```python
from build123d import *
from OCP.BRepAlgoAPI import BRepAlgoAPI_Cut
from OCP.TopTools import TopTools_ListOfShape

# Parameters (mm, degrees)
SZKIC1_W                               = 25
SZKIC1_H                               = 20
DODANIE_WYCI_GNI_CIE1_DEPTH            = 42.5
WYTNIJ_WYCI_GNI_CIE1_REACH             = 52.312
SZKIC2_R                               = 5.1
WYTNIJ_WYCI_GNI_CIE2_REACH             = 50.606
SZKIC3_R                               = 5.1
DODANIE_WYCI_GNI_CIE2_START            = -20
DODANIE_WYCI_GNI_CIE2_DEPTH            = 20
ZAOKR_GLENIE2_R                        = 0.75
SZKIC7_W                               = 25
SZKIC7_H                               = 15
DODANIE_WYCI_GNI_CIE3_DEPTH            = 2
WYTNIJ_WYCI_GNI_CIE4_REACH             = 49.817
SZKIC8_R                               = 4.05
SFAZOWANIE1_SIZE                       = 7.5
WYCI_CIE_WYCI_GNI_CIE_START            = 5.5
WYCI_CIE_WYCI_GNI_CIE_PO_CIE_CE1_DEPTH = 3
ZAOKR_GLENIE3_R                        = 2
ZAOKR_GLENIE4_START                    = -11
ZAOKR_GLENIE4_DEPTH                    = 22
ZAOKR_GLENIE3_OF_LUSTRO2_R             = 2
ZAOKR_GLENIE5_R                        = 5
ZAOKR_GLENIE6_R                        = 1
SFAZOWANIE2_SIZE                       = 1.5
WYTNIJ_WYCI_GNI_CIE5_REACH             = 52.312
SZKIC12_R                              = 5.1


with BuildPart() as part:
    # Szkic1 → Dodanie-wyciągnięcie1 (new body)
    with BuildSketch(Plane.XY):
        Rectangle(SZKIC1_W, SZKIC1_H)
    extrude(amount=DODANIE_WYCI_GNI_CIE1_DEPTH)

    # Szkic2 → Wytnij-wyciągnięcie1 (cut, up to next)
    with BuildSketch(Plane(origin=(12.5, 0, 0), x_dir=(0, 0, -1), z_dir=(1, 0, 0)), mode=Mode.PRIVATE) as wytnij_wyci_gni_cie1_sk1:
        with Locations((-8, 0)):
            Circle(SZKIC2_R)
    wytnij_wyci_gni_cie1_tool1 = extrude(wytnij_wyci_gni_cie1_sk1.sketch, amount=-WYTNIJ_WYCI_GNI_CIE1_REACH, mode=Mode.PRIVATE) & part.part
    add(wytnij_wyci_gni_cie1_tool1.solids().sort_by_distance((12.5, 0, 8))[0], mode=Mode.SUBTRACT)

    # Szkic3 → Wytnij-wyciągnięcie2 (cut, up to next)
    with BuildSketch(Plane(origin=(0, 10, 0), x_dir=(1, 0, 0), z_dir=(0, 1, 0)), mode=Mode.PRIVATE) as wytnij_wyci_gni_cie2_sk1:
        with Locations(Location((0, -19.5, 0), (0, 0, 270))):
            Circle(SZKIC3_R)
    wytnij_wyci_gni_cie2_tool1 = extrude(wytnij_wyci_gni_cie2_sk1.sketch, amount=-WYTNIJ_WYCI_GNI_CIE2_REACH, mode=Mode.PRIVATE) & part.part
    add(wytnij_wyci_gni_cie2_tool1.solids().sort_by_distance((0, 10, 19.5))[0], mode=Mode.SUBTRACT)

    # Dodanie-wyciągnięcie2: read off the stored shape, not the designer's step
    # Dodanie-wyciągnięcie2 outline → Dodanie-wyciągnięcie2 (add)
    with BuildSketch(Plane(origin=(0, 10, 0), x_dir=(1, 0, 0), z_dir=(0, 1, 0)).offset(DODANIE_WYCI_GNI_CIE2_START)):
        with BuildLine():
            Line((-12.5, 0), (-2.545584412, 0))
            ThreePointArc((-2.545584412, 0), (-4.049799766, 3.19027229), (-2.482438317, 6.35))
            Line((-2.482438317, 6.35), (-12.5, 6.35))
            Line((-12.5, 6.35), (-12.5, 0))
        make_face()
        with BuildLine():
            Line((12.5, 0), (12.5, 6.35))
            Line((12.5, 6.35), (2.482438317, 6.35))
            ThreePointArc((2.482438317, 6.35), (4.049799766, 3.19027229), (2.545584412, 0))
            Line((2.545584412, 0), (12.5, 0))
        make_face()
    extrude(amount=DODANIE_WYCI_GNI_CIE2_DEPTH)

    # Zaokrąglenie2
    zaokr_glenie2_edges = [part.edges().sort_by_distance(p)[0] for p in [
        (-2.482438317, 0, -6.35),
        (2.482438317, 0, -6.35),
    ]]
    fillet(zaokr_glenie2_edges, radius=ZAOKR_GLENIE2_R)

    # Szkic7 → Dodanie-wyciągnięcie3 (add)
    with BuildSketch(Plane.XZ.offset(10)):
        with Locations((0, 1.15)):
            Rectangle(SZKIC7_W, SZKIC7_H)
    extrude(amount=-DODANIE_WYCI_GNI_CIE3_DEPTH)

    # Szkic8 → Wytnij-wyciągnięcie4 (cut, up to next)
    with BuildSketch(Plane(origin=(0, -8, 0), x_dir=(1, 0, 0), z_dir=(0, 1, 0)), mode=Mode.PRIVATE) as wytnij_wyci_gni_cie4_sk1:
        with Locations((0, 3.15)):
            Circle(SZKIC8_R)
    wytnij_wyci_gni_cie4_tool1 = extrude(wytnij_wyci_gni_cie4_sk1.sketch, amount=WYTNIJ_WYCI_GNI_CIE4_REACH, mode=Mode.PRIVATE) & part.part
    add(wytnij_wyci_gni_cie4_tool1.solids().sort_by_distance((0, -8, -3.15))[0], mode=Mode.SUBTRACT)

    # Sfazowanie1
    sfazowanie1_edges = [part.edges().sort_by_distance(p)[0] for p in [
        (-12.5, 0, -6.35),
        (12.5, 0, -6.35),
    ]]
    chamfer(sfazowanie1_edges, length=SFAZOWANIE1_SIZE)


with BuildPart() as wyci_cie_wyci_gni_cie_po_cie_ce1_tool:
    # Wycięcie-wyciągnięcie po ścieżce1: read off the stored shape, not the designer's step
    # Wycięcie-wyciągnięcie po ścieżce1 outlin → Wycięcie-wyciągnięcie po ścieżce1 (new body)
    with BuildSketch(Plane(origin=(0, 0, 0), x_dir=(1, 0, 0), z_dir=(0, 1, 0)).offset(WYCI_CIE_WYCI_GNI_CIE_START)):
        with BuildLine():
            Line((-8.398959236, 2.951040764), (-9.601040764, 1.748959236))
            add(Edge.make_bspline(
                [(-9.601040764, 1.748959236), (-9.209595956, 0.772190109), (-8.65567701, -0.205079485), (-7.121419805, -2.018854383), (-6.15542851, -2.840889353), (-3.89496705, -4.097344098), (-2.618886758, -4.525976788), (0.018436022, -4.858092268), (1.356613032, -4.766181401), (3.844325913, -4.116700841), (4.978679647, -3.572124587), (6.907257886, -2.213562211), (7.697476445, -1.410485572), (8.875702434, 0.189942932), (9.295310391, 0.978883557), (9.600922152, 1.74907375)],
                knots=[0.044527741, 0.044527741, 0.044527741, 0.044527741, 0.163961774, 0.163961774, 0.283395806, 0.283395806, 0.402829838, 0.402829838, 0.522263871, 0.522263871, 0.641697903, 0.641697903, 0.761131935, 0.761131935, 0.869411924, 0.869411924, 0.869411924, 0.869411924], degree=3))
            Line((9.600922152, 1.74907375), (8.398612397, 2.951387603))
            add(Edge.make_bspline(
                [(-8.398959236, 2.951040764), (-8.143623085, 2.110383322), (-7.721254142, 1.22892436), (-6.543030407, -0.407961014), (-5.768609422, -1.171170966), (-3.942260695, -2.384057538), (-2.87593166, -2.830554933), (-0.670426419, -3.287743264), (0.481400093, -3.292782379), (2.627656604, -2.909796026), (3.631791424, -2.516326215), (5.35458893, -1.493813298), (6.079684963, -0.860499), (7.238136236, 0.482263814), (7.674817273, 1.192485201), (8.155489955, 2.24471168), (8.28334822, 2.593485223), (8.398612397, 2.951387603)],
                knots=[0.044527741, 0.044527741, 0.044527741, 0.044527741, 0.163961774, 0.163961774, 0.283395806, 0.283395806, 0.402829838, 0.402829838, 0.522263871, 0.522263871, 0.641697903, 0.641697903, 0.761131935, 0.761131935, 0.880565968, 0.880565968, 0.940774458, 0.940774458, 0.940774458, 0.940774458], degree=3))
        make_face()
    wyci_cie_wyci_gni_cie_po_cie_ce1 = extrude(amount=WYCI_CIE_WYCI_GNI_CIE_PO_CIE_CE1_DEPTH)


with BuildPart() as part_1:
    add(part.part)

    # Wycięcie-wyciągnięcie po ścieżce1: cut by wyci_cie_wyci_gni_cie_po_cie_ce1_tool, with a tolerance
    wyci_cie_wyci_gni_cie_po_cie_ce1_stock = TopTools_ListOfShape()
    wyci_cie_wyci_gni_cie_po_cie_ce1_stock.Append(part_1.part.wrapped)
    wyci_cie_wyci_gni_cie_po_cie_ce1_tools = TopTools_ListOfShape()
    wyci_cie_wyci_gni_cie_po_cie_ce1_tools.Append(wyci_cie_wyci_gni_cie_po_cie_ce1_tool.part.wrapped)
    wyci_cie_wyci_gni_cie_po_cie_ce1_cut = BRepAlgoAPI_Cut()
    wyci_cie_wyci_gni_cie_po_cie_ce1_cut.SetArguments(wyci_cie_wyci_gni_cie_po_cie_ce1_stock)
    wyci_cie_wyci_gni_cie_po_cie_ce1_cut.SetTools(wyci_cie_wyci_gni_cie_po_cie_ce1_tools)
    wyci_cie_wyci_gni_cie_po_cie_ce1_cut.SetFuzzyValue(0.00001)
    wyci_cie_wyci_gni_cie_po_cie_ce1_cut.Build()
    add(Compound.cast(wyci_cie_wyci_gni_cie_po_cie_ce1_cut.Shape()).solids(), mode=Mode.REPLACE)

    # Zaokrąglenie3
    zaokr_glenie3_edges = [part_1.edges().sort_by_distance(p)[0] for p in [
        (-8.398959236, 7, -2.951040764),
        (8.398612397, 7, -2.951387603),
    ]]
    fillet(zaokr_glenie3_edges, radius=ZAOKR_GLENIE3_R)

    # Zaokrąglenie4: read off the stored shape, not the designer's step
    # Zaokrąglenie4 outline → Zaokrąglenie4 (cut)
    with BuildSketch(Plane(origin=(0, 0, 0), x_dir=(1, 0, 0), z_dir=(0, 1, 0)).offset(ZAOKR_GLENIE4_START)):
        with BuildLine():
            Line((5, 6.35), (3.757359313, 6.35))
            ThreePointArc((3.757359313, 6.35), (4.90540961, 6.121638598), (5.878679656, 5.471320344))
            Line((5.878679656, 5.471320344), (5, 6.35))
        make_face()
        with BuildLine():
            ThreePointArc((-5.878679656, 5.471320344), (-4.90540961, 6.121638598), (-3.757359313, 6.35))
            Line((-3.757359313, 6.35), (-5, 6.35))
            Line((-5, 6.35), (-5.878679656, 5.471320344))
        make_face()
    extrude(amount=ZAOKR_GLENIE4_DEPTH, mode=Mode.SUBTRACT)

    # Lustro2: Wycięcie-wyciągnięcie po ścieżce1 across plane
    add(wyci_cie_wyci_gni_cie_po_cie_ce1.mirror(Plane.ZX), mode=Mode.SUBTRACT)

    # Zaokrąglenie3 of Lustro2
    zaokr_glenie3_of_lustro2_edges = [part_1.edges().sort_by_distance(p)[0] for p in [
        (-8.398959236, -7, -2.951040764),
        (8.398612397, -7, -2.951387603),
    ]]
    fillet(zaokr_glenie3_of_lustro2_edges, radius=ZAOKR_GLENIE3_OF_LUSTRO2_R)

    # Zaokrąglenie5
    # the kernel refuses this fillet: 5 mm, written as the material it takes off along each edge
    with BuildSketch(Plane(origin=(-12.5, 15.17766953, 1.15), x_dir=(0.7071067811865477, 0, -0.7071067811865472), z_dir=(0, -1, 0)), Plane(origin=(12.5, -15.17766953, 1.15), x_dir=(-0.7071067811865474, 0, -0.7071067811865476), z_dir=(0, 1, 0))) as zaokr_glenie5_piece_1:
        with BuildLine():
            CenterArc((ZAOKR_GLENIE5_R * 0.414213562373, ZAOKR_GLENIE5_R), ZAOKR_GLENIE5_R, 225, 45)
            Line((-ZAOKR_GLENIE5_R * 0.292893218813, ZAOKR_GLENIE5_R * 0.292893218813), (0, 0))
            Line((0, 0), (ZAOKR_GLENIE5_R * 0.414213562373, 0))
        make_face()
    extrude(amount=30.355339059, mode=Mode.SUBTRACT)

    # Zaokrąglenie6
    zaokr_glenie6_edges = [part_1.edges().sort_by_distance(p)[0] for p in [
        (-8.457106781, 10, -2.892893219),
        (-5.01866332, 10, -6.071968443),
        (5.01866332, 10, -6.071968443),
        (8.457106781, 10, -2.892893219),
        (12.119397663, 10, 1.30765065),
        (-12.119397663, 10, 1.30765065),
        (-12.5, 10, 22.860533906),
        (12.5, 10, 22.860533906),
    ]]
    fillet(zaokr_glenie6_edges, radius=ZAOKR_GLENIE6_R)

    # Sfazowanie2
    # the kernel refuses this chamfer: 1.5 mm, written as the material it takes off along each edge
    with BuildSketch(Plane(origin=(1e-09, 10, -3.15), x_dir=(0.08224322624349094, 0, -0.9966122875707795), z_dir=(-0.9966122875707795, 0, -0.08224322624349094))) as sfazowanie2_piece_1:
        Polygon((4.049999999 + SFAZOWANIE2_SIZE, 0), (4.049999999, SFAZOWANIE2_SIZE), (4.049999999, 0), align=None)
    revolve(axis=Axis((1e-09, 10, -3.15), (0, -1, 0)), revolution_arc=136.340040588, mode=Mode.SUBTRACT)
    with BuildSketch(Plane(origin=(-1e-09, 10, -3.15), x_dir=(-0.6285393608328834, 0, 0.7777777779570398), z_dir=(0.7777777779570398, 0, 0.6285393608328834))) as sfazowanie2_piece_2:
        Polygon((4.049999999 + SFAZOWANIE2_SIZE, 0), (4.049999999, SFAZOWANIE2_SIZE), (4.049999999, 0), align=None)
    revolve(axis=Axis((-1e-09, 10, -3.15), (0, -1, 0)), revolution_arc=136.340040588, mode=Mode.SUBTRACT)
    with BuildSketch(Plane(origin=(0, 10, -3.15), x_dir=(0.6285393610141453, 0, 0.7777777778105581), z_dir=(0.7777777778105581, 0, -0.6285393610141453))) as sfazowanie2_piece_3:
        Polygon((4.05 + SFAZOWANIE2_SIZE, 0), (4.05, SFAZOWANIE2_SIZE), (4.05, 0), align=None)
    revolve(axis=Axis((0, 10, -3.15), (0, -1, 0)), revolution_arc=77.884882532, mode=Mode.SUBTRACT)

    # Szkic12 → Wytnij-wyciągnięcie5 (cut, up to next)
    with BuildSketch(Plane.ZY.offset(12.5), mode=Mode.PRIVATE) as wytnij_wyci_gni_cie5_sk1:
        with Locations((32.5, 0)):
            Circle(SZKIC12_R)
    wytnij_wyci_gni_cie5_tool1 = extrude(wytnij_wyci_gni_cie5_sk1.sketch, amount=-WYTNIJ_WYCI_GNI_CIE5_REACH, mode=Mode.PRIVATE) & part_1.part
    add(wytnij_wyci_gni_cie5_tool1.solids().sort_by_distance((-12.5, 0, 32.5))[0], mode=Mode.SUBTRACT)


solid = part_1.part
```
CAD build for the part. Positions are in the model's coordinates, mm. A direction names the side the tool comes from. Round coordinates to 2 decimals unless told otherwise and drop trailing zeros. Order: outer loops, then holes, each group sorted by start corner. A loop starts at its lowest first (then second) coordinate and runs counter-clockwise, first axis right, second up. Notation, with made-up numbers: (-1.5, 16) - (29.5, 16) arc R29 ccw to (29.5, 41) - close; hole circle Ø5 at (87.25, 77). An arc over 180 degrees is marked (long way). Answer as CSV lines item,"result". Start each with the question number.
1. Saw through at D-D, the plane z = 19.5. Write the cut outline in (x, y).
2. Tool access for faces 5 (the face through (1.532, 0.14, 24.364)), 6 (the face through (0, 8.5, 3.4)), 7 (the face through (3.443, 0.809, -5.907)): list every direction of +Z, -Z, +X, -X, +Y, -Y with a clear straight run to the whole face (end or side of a thin tool).
3. Saw through at A-A, the plane z = 32.5. Write the cut outline in (x, y).
4. Pull direction X, two halves, no side cores. Call faces 1 (the face through (0, -8, -3)), 2 (the face through (12.5, -1, 23)), 3 (the face through (-12.215, 9.699, 23.135)), 4 (the face through (0, -9, -6.35)): +X half, -X half, draft (parallel to the pull), parting line (faces both ways), or undercut.
5. Saw through at B-B, the plane y = 3.5. Write the cut outline in (x, z), and give its area (3 significant figures).
6. Drill centre lines: L1, parallel to Y at x = 3.75, z = 8; L2, parallel to Z at x = -6, y = 0.25; L3, parallel to Z at x = -0.75, y = 2.5. Where is each one in solid material? Low to high. Write a range as [from, to].
7. Saw through at C-C, the plane x = 0. Count the separate pieces of the cut face and the enclosed holes in it, and give its area (3 significant figures).
8. Pin check, flat tips, straight feed: pin 1 (2 mm diameter, centred on x = 1.5, z = -1.5, fed in from +Y); pin 2 (11.5 mm diameter, centred on y = 0, z = 8, fed in from -X); pin 3 (4 mm diameter, centred on x = 9.5, y = 6, fed in from -Z); pin 4 (1.5 mm diameter, centred on x = 0, y = 1, fed in from -Z). Stop position of each tip, or through.
Model answer:
1,outline,"(-12.5, -10) - (-5.1, -10) - (-5.1, 10) - (-11.5, 10) arc R1 ccw to (-12.5, 9) - close; (5.1, -10) - (12.5, -10) - (12.5, 9) arc R1 ccw to (11.5, 10) - (5.1, 10) - close"
2,face 5,"+Y, -Y"
2,face 6,"none"
2,face 7,"+Y"
3,outline,"(-12.5, -10) - (12.5, -10) - (12.5, -5.1) - (-12.5, -5.1) - close; (-12.5, 5.1) - (12.5, 5.1) - (12.5, 9) arc R1 ccw to (11.5, 10) - (-11.5, 10) arc R1 ccw to (-12.5, 9) - close"
4,face 1,"undercut"
4,face 2,"+X half"
4,face 3,"-X half"
4,face 4,"draft"
5,outline,"(-12.5, 3.22) arc R5 ccw to (-11.04, -0.31) - (-5.88, -5.47) arc R3 ccw to (-4, -6.34) arc R0.75 ccw to (-3.48, -5.22) arc R4.05 cw (long way) to (3.48, -5.22) arc R0.75 ccw to (4, -6.34) arc R3 ccw to (5.88, -5.47) - (11.04, -0.31) arc R5 ccw to (12.5, 3.22) - (12.5, 4.29) - (-12.5, 4.29) - close; (-12.5, 11.71) - (12.5, 11.71) - (12.5, 28.79) - (-12.5, 28.79) - close; (-12.5, 36.21) - (12.5, 36.21) - (12.5, 42.5) - (-12.5, 42.5) - close; hole circle Ø10.2 at (0, 19.5)"
5,area,"661 mm²"
6,L1,"y = [-10, -5.1], [5.1, 10]"
6,L2,"z = [-5.35, 2.91], [13.09, 27.41], [37.59, 42.5]"
6,L3,"z = [0.83, 3.55], [12.45, 14.46], [24.54, 28.05], [36.95, 42.5]"
7,separate pieces,"2"
7,enclosed holes,"4"
7,area,"469 mm²"
8,pin 1,"stops at y = -8"
8,pin 2,"stops at x = -12.5"
8,pin 3,"stops at z = -3.85"
8,pin 4,"stops at z = 0.83"
